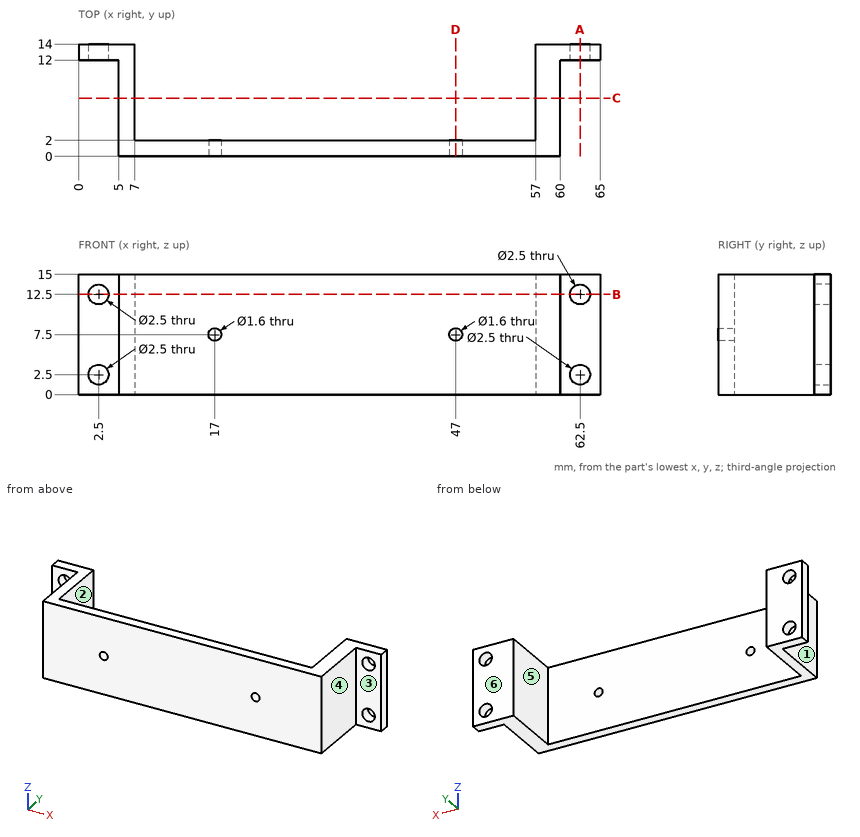
Can you work these out from the drawing? Everything is in mm from the part's minimum corner. A direction names the side the tool comes from. Round coordinates to 2 decimals unless told otherwise and drop trailing zeros. Loops run counter-clockwise (first coordinate to the right, second up) from the corner with the lowest first, then second, coordinate; pieces in that order, holes last. Notation, with made-up numbers: M 29.25,-28.5 L 35.25,-28.5 A18 ccw 35.25,-0.5 Z; hole C 84.25,58.25 d11. An arc over 180 degrees is marked long. Answer in a Markdown table with one row per item.
1. I'm going to push flat-ended pins straight in: pin 1 Ø1.5 at (x, z) = (34, 3.5) entering from +Y; pin 2 Ø6 at (y, z) = (7.5, 10.5) entering from -X; pin 3 Ø4 at (x, z) = (2.5, 12.5) entering from -Y. Where does each tip first touch, or does it pass through?
Established:
| item | result |
|---|---|
| pin 1 | y = 2 |
| pin 2 | x = 5 |
| pin 3 | y = 12 |
2. If we section it at C-C, the plane y = 7.25: Please give me the cut outline in (x, z).
Established:
| item | result |
|---|---|
| outline | M 5,0 L 7,0 L 7,15 L 5,15 Z; M 57,0 L 60,0 L 60,15 L 57,15 Z |
3. On a 3-axis mill with a long thin cutter (end or side, diameter ignored), from which of +Z, -Z, +X, -X, +Y, -Y can I reach the whole of each face in a straight line? I mean the marked faces 5 and 6. Say none if no direction works.
Established:
| item | result |
|---|---|
| face 5 | +Z, -Z, +Y |
| face 6 | +Z, -Z, +X, -X, +Y |
4. Thinking about a two-plate mould opening in X: for the marked faces 1, 2, 3 and 4, which applies, pulls with the +X half, pulls with the -X half, needs draft (parallel to the pull), parting line crosses it, or undercut?
Established:
| item | result |
|---|---|
| face 1 | pulls with the -X half |
| face 2 | undercut |
| face 3 | needs draft |
| face 4 | pulls with the +X half |
5. If we section it at D-D, the plane x = 47: Please give me the cut outline in (y, z), plus the area to 3 significant figures.
Established:
| item | result |
|---|---|
| outline | M 0,0 L 2,0 L 2,6.7 L 0,6.7 Z; M 0,8.3 L 2,8.3 L 2,15 L 0,15 Z |
| area | 26.8 mm² |
6. If we section it at A-A, the plane x = 62.5: Please give me the cut outline in (y, z), plus the area to 3 significant figures.
Established:
| item | result |
|---|---|
| outline | M 12,0 L 14,0 L 14,1.25 L 12,1.25 Z; M 12,3.75 L 14,3.75 L 14,11.25 L 12,11.25 Z; M 12,13.75 L 14,13.75 L 14,15 L 12,15 Z |
| area | 20.0 mm² |
7. If we section it at B-B, the plane z = 12.5: Please give me the cut outline in (x, y), plus the area to 3 significant figures.
Established:
| item | result |
|---|---|
| outline | M 0,12 L 1.25,12 L 1.25,14 L 0,14 Z; M 3.75,12 L 5,12 L 5,0 L 60,0 L 60,12 L 61.25,12 L 61.25,14 L 57,14 L 57,2 L 7,2 L 7,14 L 3.75,14 Z; M 63.75,12 L 65,12 L 65,14 L 63.75,14 Z |
| area | 180 mm² |
8. Please list where these lines run through material, in increasing order: line 1 (X direction, y = 13.4, z = 2.5); line 2 (X direction, y = 0.8, z = 7.5); line 3 (Z direction, x = 47, y = 1.3). Write a range as from..to.
Established:
| item | result |
|---|---|
| line 1 | 0..1.25, 3.75..7, 57..61.25, 63.75..65 |
| line 2 | 5..16.2, 17.8..46.2, 47.8..60 |
| line 3 | 0..6.7, 8.3..15 |
